from build123d import *

# Parameters (mm, degrees)
F0_W     = 50.8
F0_H     = 27.94
F1_DEPTH = 2.54
F2_R     = 3.81
F4_DEPTH = 2.54


with BuildPart() as f1:
    # F0 (on Top) → F1 (new body)
    with BuildSketch(Plane.XY):
        Rectangle(F0_W, F0_H)
    extrude(amount=F1_DEPTH)

    # F2
    f2_edges = [f1.edges().sort_by_distance(p)[0] for p in [
        (-25.4, 13.97, 1.27),
        (25.4, 13.97, 1.27),
        (-25.4, -13.97, 1.27),
        (25.4, -13.97, 1.27),
    ]]
    fillet(f2_edges, radius=F2_R)

    # F3 (on face) → F4 (join)
    with BuildSketch(Plane.XY.offset(2.54)):
        with BuildLine():
            Line((-18.796, -11.176), (18.796, -11.176))
            ThreePointArc((18.796, -11.176), (21.490077, -10.060077), (22.606, -7.366))
            Line((22.606, -7.366), (22.606, 7.366))
            ThreePointArc((22.606, 7.366), (21.490077, 10.060077), (18.796, 11.176))
            Line((18.796, 11.176), (-18.796, 11.176))
            ThreePointArc((-18.796, 11.176), (-21.490077, 10.060077), (-22.606, 7.366))
            Line((-22.606, 7.366), (-22.606, -7.366))
            ThreePointArc((-22.606, -7.366), (-21.490077, -10.060077), (-18.796, -11.176))
        make_face()
        with BuildLine():
            ThreePointArc((18.796, 9.906), (20.592051, 9.162051), (21.336, 7.366))
            Line((21.336, 7.366), (21.336, -7.366))
            ThreePointArc((21.336, -7.366), (20.592051, -9.162051), (18.796, -9.906))
            Line((18.796, -9.906), (-18.796, -9.906))
            ThreePointArc((-18.796, -9.906), (-20.592051, -9.162051), (-21.336, -7.366))
            Line((-21.336, -7.366), (-21.336, 7.366))
            ThreePointArc((-21.336, 7.366), (-20.592051, 9.162051), (-18.796, 9.906))
            Line((-18.796, 9.906), (18.796, 9.906))
        make_face(mode=Mode.SUBTRACT)
    extrude(amount=F4_DEPTH)


solid = f1.part
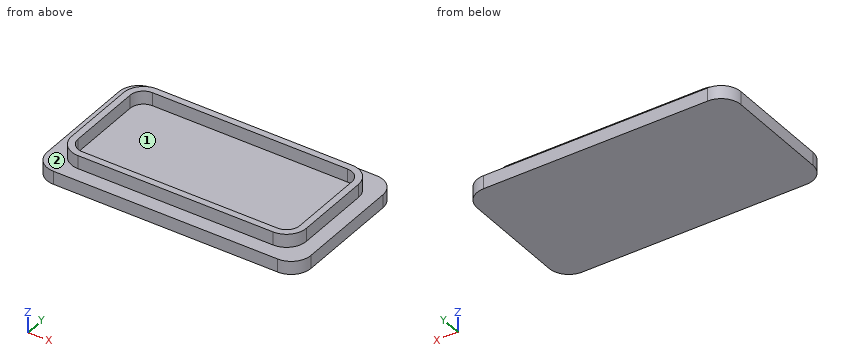
Model file for the job. Use its own axes, mm. Face numbers are marked on the shaded views. Give positions to 0.01 mm unless a question says otherwise; leave off trailing zeros. Order: outer loops, then holes, each group sorted by start corner. A loop starts at its lowest first (then second) coordinate and runs counter-clockwise, first axis right, second up. Notation, with made-up numbers: (79.25, -24) - (105.25, -24) arc R13 ccw to (105.25, -5) - close; hole circle Ø10 at (71, 27). An arc over 180 degrees is marked (long way). Write item = value, one per line. Start each with the question number.
1. Probe line 1 along X through (y, z) = (-3, 4.55); line 2 along Y through (x, z) = (15.5, 3.65); line 3 along Z through (x, y) = (-1, 4.5). List the from-to ranges inside material, lowest first.
2. Two-plate mould, pull along Y, no slides. Class the marked faces 1 and 2: pulls with the +Y half, pulls with the -Y half, needs draft (parallel to the pull), parting line crosses it, or undercut.
3. Drop flat-ended pins along their axis: P1, Ø0.8, axis at x = 2, z = 4, coming from the +Y side; P2, Ø2, axis at y = 3.5, z = 3.5, coming from the +X side; P3, Ø6, axis at x = 7.5, y = 4.5, coming from the +Z side; P4, Ø0.8, axis at y = -1, z = 3.5, coming from the -X side. Give the stop position or say it passes through.
4. Cut at A-A, the plane z = 3.9. List the corners of the cut face in (x, y).
5. Cut at B-B, the plane y = 0.25. List the corners of the cut face in (x, z), and give its area (3 significant figures).
6. Cut at C-C, the plane x = -1. List the corners of the cut face in (y, z).
Taken from the geometry:
q1.line_1 = -22.61 to -21.34, 21.34 to 22.61
q1.line_2 = -11.18 to -9.91, 9.91 to 11.18
q1.line_3 = 0 to 2.54
q2.face_1 = undercut
q2.face_2 = needs draft
q3.P1 = 11.18
q3.P2 = 25.4
q3.P3 = 2.54
q3.P4 = -22.61
q4.outline = (-22.61, -7.37) arc R3.81 ccw to (-18.8, -11.18) - (18.8, -11.18) arc R3.81 ccw to (22.61, -7.37) - (22.61, 7.37) arc R3.81 ccw to (18.8, 11.18) - (-18.8, 11.18) arc R3.81 ccw to (-22.61, 7.37) - close; hole (-21.34, -7.37) arc R2.54 ccw to (-18.8, -9.91) - (18.8, -9.91) arc R2.54 ccw to (21.34, -7.37) - (21.34, 7.37) arc R2.54 ccw to (18.8, 9.91) - (-18.8, 9.91) arc R2.54 ccw to (-21.34, 7.37) - close
q5.outline = (-25.4, 0) - (25.4, 0) - (25.4, 2.54) - (22.61, 2.54) - (22.61, 5.08) - (21.34, 5.08) - (21.34, 2.54) - (-21.34, 2.54) - (-21.34, 5.08) - (-22.61, 5.08) - (-22.61, 2.54) - (-25.4, 2.54) - close
q5.area = 135 mm²
q6.outline = (-13.97, 0) - (13.97, 0) - (13.97, 2.54) - (11.18, 2.54) - (11.18, 5.08) - (9.91, 5.08) - (9.91, 2.54) - (-9.91, 2.54) - (-9.91, 5.08) - (-11.18, 5.08) - (-11.18, 2.54) - (-13.97, 2.54) - close
